Read the model definition and answer for the solid it produces. Units are mm, in the model's axes. Face numbers are marked on the shaded views. A direction names the side the tool comes from. Coordinates: 2 decimals unless noted, no trailing zeros. Write each loop counter-clockwise with the first axis right and the second up, starting at its lowest first coordinate (ties: lowest second). Pieces come first, ordered by that corner, then holes.
(1) The mould has two halves that part along Y. Classify the marked faces 1, 2, 3 and 4: +Y half, -Y half, draft (parallel to the pull), parting line (faces both ways), or undercut.
(2) Which of the six approach directions +Z, -Z, +X, -X, +Y, -Y give full straight-line access (tool end or side, diameter ignored) to the marked faces 5, 6 and 7?
(3) Section C-C on x = 33.5 is taken. Write down the section's boundary in (y, z).
(4) Given pin 1 (8 mm diameter, centred on x = 46, z = 19.5, fed in from +Y); pin 2 (4 mm diameter, centred on x = 43.5, z = 6, fed in from +Y); pin 3 (4 mm diameter, centred on y = 22.5, z = 11.5, fed in from -X); pin 4 (5 mm diameter, centred on x = 57.15, y = 31.75, fed in from -Z), each flat-ended and moving along its own axis, determine where each tip first touches the part or whether it passes through.
(5) Section D-D on y = 14.5 is taken. Write down the section's boundary in (x, z), then the cut area to 3 significant figures.
(6) Section A-A on x = 6.35 is taken. Write down the section's boundary in (y, z) (3 decimals).
(7) Find the intervals of material crossed by probe 1 along X at (y, z) = (31.75, 5.5) (3 decimals); probe 2 along X at (y, z) = (57.15, 7.75) (3 decimals), in increasing order.
from build123d import *

# Parameters (mm, degrees)
F0_W     = 63.5
F0_H     = 63.5
F1_DEPTH = 25.4
F2_W     = 63.5
F2_H     = 63.5
F3_DEPTH = 12.7
F5_DEPTH = 25.4
F7_DEPTH = 25.4
F8_R     = 31.74999
F9_R     = 19.04999


# Not quite as in the source:
# - a fillet or chamfer is up to 0.001 mm smaller than in the source, because OpenCascade refuses the exact size


with BuildPart() as f1:
    # F0 (on Top) → F1 (new body)
    with BuildSketch(Plane.XY):
        with Locations((31.75, 31.75)):
            Rectangle(F0_W, F0_H)
    extrude(amount=F1_DEPTH)

    # F2 (on face) → F3 (cut)
    with BuildSketch(Plane.XY.offset(25.4)):
        with Locations((31.75, 31.75)):
            Rectangle(F2_W, F2_H)
        Polygon((12.7, 50.8), (31.75, 50.8), (50.8, 50.8), (50.8, 31.75), (50.8, 12.7), (12.7, 12.7), align=None, mode=Mode.SUBTRACT)
    extrude(amount=-F3_DEPTH, mode=Mode.SUBTRACT)

    # F4 (on face) → F5 (cut)
    with BuildSketch(Plane.XY.offset(12.7)):
        with BuildLine():
            ThreePointArc((8.333406776, 34.22925847), (4.9746257807, 34.6116377753), (3.175, 31.75))
            Line((3.175, 31.75), (6.35, 31.75))
            Line((6.35, 31.75), (8.333406776, 34.22925847))
        make_face()
        with BuildLine():
            ThreePointArc((34.925, 57.15), (33.9950640303, 59.3950640303), (31.75, 60.325))
            ThreePointArc((31.75, 60.325), (29.5049359697, 54.9049359697), (34.925, 57.15))
        make_face()
        with BuildLine():
            Line((6.35, 31.75), (3.175, 31.75))
            ThreePointArc((3.175, 31.75), (6.35, 28.575), (9.525, 31.75))
            ThreePointArc((9.525, 31.75), (9.2116377753, 33.1253742193), (8.333406776, 34.22925847))
            Line((8.333406776, 34.22925847), (6.35, 31.75))
        make_face()
        with BuildLine():
            ThreePointArc((55.166593224, 29.27074153), (58.5253742193, 28.8883622247), (60.325, 31.75))
            Line((60.325, 31.75), (57.15, 31.75))
            Line((57.15, 31.75), (55.166593224, 29.27074153))
        make_face()
        with BuildLine():
            Line((57.15, 31.75), (60.325, 31.75))
            ThreePointArc((60.325, 31.75), (55.7746257807, 34.6116377753), (55.166593224, 29.27074153))
            Line((55.166593224, 29.27074153), (57.15, 31.75))
        make_face()
        with BuildLine():
            ThreePointArc((34.925, 6.35), (29.5049359697, 8.5950640303), (31.75, 3.175))
            ThreePointArc((31.75, 3.175), (33.9950640303, 4.1049359697), (34.925, 6.35))
        make_face()
    extrude(amount=-F5_DEPTH, mode=Mode.SUBTRACT)

    # F6 (on face) → F7 (cut)
    with BuildSketch(Plane.XY.offset(25.4)):
        with BuildLine():
            ThreePointArc((41.275, 31.75), (38.4851920908, 38.4851920908), (31.75, 41.275))
            Line((31.75, 41.275), (31.75, 22.225))
            ThreePointArc((31.75, 22.225), (38.4851920908, 25.0148079092), (41.275, 31.75))
        make_face()
        with BuildLine():
            Line((31.75, 22.225), (31.75, 41.275))
            ThreePointArc((31.75, 41.275), (22.225, 31.75), (31.75, 22.225))
        make_face()
    extrude(amount=-F7_DEPTH, mode=Mode.SUBTRACT)

    # F8 (radius 31.75 in the source; OpenCascade refuses exactly that, so slightly less here)
    f8_edges = [f1.edges().sort_by_distance(p)[0] for p in [
        (0, 0, 6.35),
        (63.5, 0, 6.35),
        (63.5, 63.5, 6.35),
        (0, 63.5, 6.35),
    ]]
    fillet(f8_edges, radius=F8_R)

    # F9 (radius 19.05 in the source; OpenCascade refuses exactly that, so slightly less here)
    f9_edges = [f1.edges().sort_by_distance(p)[0] for p in [
        (12.7, 12.7, 19.05),
        (50.8, 12.7, 19.05),
        (12.7, 50.8, 19.05),
        (50.8, 50.8, 19.05),
    ]]
    fillet(f9_edges, radius=F9_R)


solid = f1.part
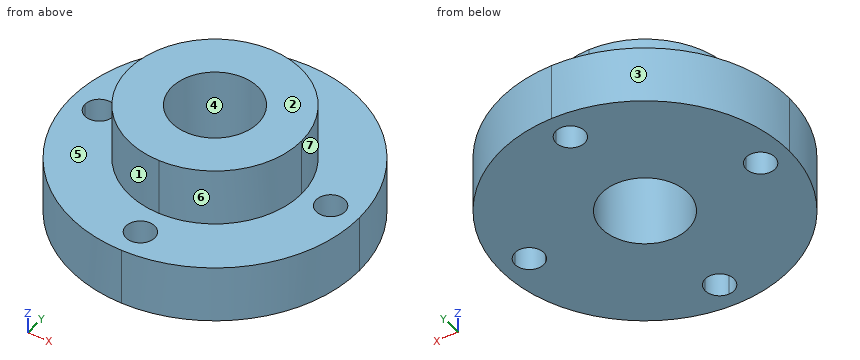
Response:
1. face 1: -Y half
1. face 2: draft
1. face 3: +Y half
1. face 4: undercut
2. face 5: +Z
2. face 6: +Z, +X, -Y
2. face 7: +Z, +X, +Y
3. outline: (0.05, 0) - (3.7, 0) - (3.7, 12.7) - (0.05, 12.7) - close; (9, 0) - (22.39, 0) - (22.39, 25.4) - (12.78, 25.4) - (12.78, 12.7) - (9, 12.7) - close; (41.11, 0) - (54.5, 0) - (54.5, 12.7) - (50.72, 12.7) - (50.72, 25.4) - (41.11, 25.4) - close; (59.8, 0) - (63.45, 0) - (63.45, 12.7) - (59.8, 12.7) - close
4. pin 1: stops at y = 47.81
4. pin 2: stops at y = 61.97
4. pin 3: stops at x = 0.84
4. pin 4: passes through
5. outline: (5.09, 0) - (58.41, 0) - (58.41, 12.7) - (39.83, 12.7) - (39.83, 25.4) - (23.67, 25.4) - (23.67, 12.7) - (5.09, 12.7) - close
5. area: 882 mm2
6. outline: (12.7, 0) - (28.575, 0) - (28.575, 12.7) - (12.7, 12.7) - close; (34.925, 0) - (50.8, 0) - (50.8, 12.7) - (34.925, 12.7) - close
7. probe 1: x = 0 to 3.175, 9.525 to 22.225, 41.275 to 53.975, 60.325 to 63.5
7. probe 2: x = 12.7 to 28.575, 34.925 to 50.8
